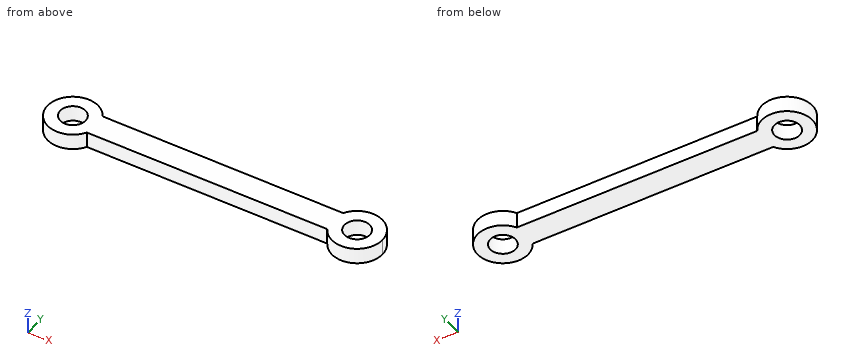
```python
from build123d import *

# Parameters (mm, degrees)
BOSS_EXTRUDE1_DEPTH = 3.175
SKETCH2_R           = 2.54
CUT_EXTRUDE1_DEPTH  = 63.775137794


with BuildPart() as part:
    # Sketch1 → Boss-Extrude1 (new body)
    with BuildSketch(Plane.XY):
        with BuildLine():
            Line((0, 5.08), (0, 0))
            Line((0, 0), (4.399409051, 0))
            ThreePointArc((4.399409051, 0), (4.906903198, 1.225199251), (5.08, 2.54))
            ThreePointArc((5.08, 2.54), (4.906903198, 3.854800749), (4.399409051, 5.08))
            Line((4.399409051, 5.08), (0, 5.08))
        make_face()
        with BuildLine():
            Line((4.399409051, 0), (0, 0))
            Line((0, 0), (0, 5.08))
            Line((0, 5.08), (4.399409051, 5.08))
            ThreePointArc((4.399409051, 5.08), (-5.08, 2.54), (4.399409051, 0))
        make_face()
        with BuildLine():
            ThreePointArc((5.08, 2.54), (4.906903198, 1.225199251), (4.399409051, 0))
            Line((4.399409051, 0), (52.750590949, 0))
            ThreePointArc((52.750590949, 0), (52.07, 2.54), (52.750590949, 5.08))
            Line((52.750590949, 5.08), (4.399409051, 5.08))
            ThreePointArc((4.399409051, 5.08), (4.906903198, 3.854800749), (5.08, 2.54))
        make_face()
        with BuildLine():
            ThreePointArc((52.750590949, 5.08), (52.07, 2.54), (52.750590949, 0))
            Line((52.750590949, 0), (57.15, 0))
            Line((57.15, 0), (57.15, 5.08))
            Line((57.15, 5.08), (52.750590949, 5.08))
        make_face()
        with BuildLine():
            Line((57.15, 0), (52.750590949, 0))
            ThreePointArc((52.750590949, 0), (58.464800749, -2.366903198), (62.23, 2.54))
            ThreePointArc((62.23, 2.54), (58.464800749, 7.446903198), (52.750590949, 5.08))
            Line((52.750590949, 5.08), (57.15, 5.08))
            Line((57.15, 5.08), (57.15, 0))
        make_face()
    extrude(amount=BOSS_EXTRUDE1_DEPTH)

    # Sketch2 → Cut-Extrude1 (cut, through all)
    with BuildSketch(Plane.XY.offset(3.175)):
        with Locations((0, 2.54)):
            Circle(SKETCH2_R)
        with Locations((57.15, 2.54)):
            Circle(SKETCH2_R)
    extrude(amount=-CUT_EXTRUDE1_DEPTH, mode=Mode.SUBTRACT)


solid = part.part
```
CAD build for the part. Positions are in the model's coordinates, mm. Coordinates: 2 decimals unless noted, no trailing zeros. Order: outer loops, then holes, each group sorted by start corner. A loop starts at its lowest first (then second) coordinate and runs counter-clockwise, first axis right, second up. Notation, with made-up numbers: (-38.75, 77.25) - (-0.75, 77.25) arc R28 ccw to (-0.75, 104.25) - close; hole circle Ø9 at (-26.75, -37). An arc over 180 degrees is marked (long way). Answer in a Markdown table with one row per item.
1. Slice it at A-A, the plane x = 0. List the corners of the cut face in (y, z) (3 decimals).
Answer:
| item | result |
|---|---|
| outline | (-2.54, 0) - (0, 0) - (0, 3.175) - (-2.54, 3.175) - close; (5.08, 0) - (7.62, 0) - (7.62, 3.175) - (5.08, 3.175) - close |
2. Slice it at D-D, the plane y = 1. List the corners of the cut face in (x, z) (3 decimals).
Answer:
| item | result |
|---|---|
| outline | (-4.841, 0) - (-2.02, 0) - (-2.02, 3.175) - (-4.841, 3.175) - close; (2.02, 0) - (55.13, 0) - (55.13, 3.175) - (2.02, 3.175) - close; (59.17, 0) - (61.991, 0) - (61.991, 3.175) - (59.17, 3.175) - close |
3. Slice it at B-B, the plane y = 6.25. List the corners of the cut face in (x, z) (3 decimals), then the cut area to 3 significant figures.
Answer:
| item | result |
|---|---|
| outline | (-3.47, 0) - (3.47, 0) - (3.47, 3.175) - (-3.47, 3.175) - close; (53.68, 0) - (60.62, 0) - (60.62, 3.175) - (53.68, 3.175) - close |
| area | 44.1 mm² |
4. Slice it at C-C, the plane z = 0.9. List the corners of the cut face in (x, y), then the cut area to 3 significant figures.
Answer:
| item | result |
|---|---|
| outline | (4.4, 0) - (52.75, 0) arc R5.08 ccw (long way) to (52.75, 5.08) - (4.4, 5.08) arc R5.08 ccw (long way) to start; hole circle Ø5.08 at (0, 2.54); hole circle Ø5.08 at (57.15, 2.54) |
| area | 363 mm² |
5. Flat gauge pins, fed straight in: P1, Ø1, axis at x = 39.5, z = 2, coming from the -Y side; P2, Ø1, axis at y = 0.5, z = 2.5, coming from the +X side. Where does each tip first touch, or does it go through?
Answer:
| item | result |
|---|---|
| P1 | y = 0 |
| P2 | x = 61.99 |
6. Drill centre lines: L1, parallel to Y at x = 0, z = 0.95; L2, parallel to X at y = 2, z = 0.7; L3, parallel to X at y = 1.75, z = 2.6. Where is each one in solid material? Low to high. Write a range as from..to.
Answer:
| item | result |
|---|---|
| L1 | -2.54..0, 5.08..7.62 |
| L2 | -5.05..-2.48, 2.48..54.67, 59.63..62.2 |
| L3 | -5.02..-2.41, 2.41..54.74, 59.56..62.17 |
